Can you work these out from the model? Positions are in its coordinate system, mm. A direction names the side the tool comes from. Give positions to 0.01 mm unless a question says otherwise; leave off trailing zeros. Loops run counter-clockwise (first coordinate to the right, second up) from the corner with the lowest first, then second, coordinate; pieces in that order, holes last. Notation, with made-up numbers: (-36, 54) - (14, 54) arc R13 ccw to (14, 72) - close; hole circle Ø8 at (17.25, 53.5). An arc over 180 degrees is marked (long way). Write item = value, one per line.
from build123d import *

# Parameters (mm, degrees)
EXTRUDE_1_DEPTH        = 16
EXTRUDE_2_DEPTH        = 12
EXTRUDE_3_DEPTH        = 20
CUT_EXTRUDE_START      = -7
CUT_EXTRUDE_1_DEPTH    = 7
SKETCH_6_R             = 10
CUT_EXTRUDE_2_DEPTH    = 71.149839629
SKETCH_7_R             = 14
CUT_EXTRUDE_3_DEPTH    = 8
HOLE_WIZARD_M8_1_D     = 6.8
HOLE_WIZARD_M8_1_DEPTH = 16.25
HOLE_WIZARD_M8_1_TIP   = 2.042926105
CUT_EXTRUDE_4_DEPTH    = 84.868945385
FILLET_3_R             = 2
FILLET_6_R             = 5


with BuildPart() as part:
    # 草图1 → 凸台-拉伸1 (new body)
    with BuildSketch(Plane(origin=(0, 0, 0), x_dir=(1, 0, 0), z_dir=(0, 1, 0))):
        with BuildLine():
            Line((40, 5), (-40, 5))
            Line((-40, 5), (-40, 0))
            ThreePointArc((-40, 0), (0, -40), (40, 0))
            Line((40, 0), (40, 5))
        make_face()
    extrude(amount=EXTRUDE_1_DEPTH)

    # 草图3 → 凸台-拉伸2 (add)
    with BuildSketch(Plane(origin=(0, 16, 0), x_dir=(1, 0, 0), z_dir=(0, 1, 0))):
        with BuildLine():
            Line((-24, 5), (-24, 0))
            ThreePointArc((-24, 0), (0, -24), (24, 0))
            Line((24, 0), (24, 5))
            Line((24, 5), (-24, 5))
        make_face()
    extrude(amount=EXTRUDE_2_DEPTH)

    # 草图4 → 凸台-拉伸3 (add)
    with BuildSketch(Plane(origin=(0, 0, -5), x_dir=(-1, 0, 0), z_dir=(0, 0, -1))):
        with BuildLine():
            Line((-45, 23), (-45, -8))
            Line((-45, -8), (-40, -8))
            Line((-40, -8), (-40, 0))
            Line((-40, 0), (40, 0))
            Line((40, 0), (40, -8))
            Line((40, -8), (45, -8))
            Line((45, -8), (45, 23))
            ThreePointArc((45, 23), (43.535533906, 26.535533906), (40, 28))
            Line((40, 28), (-40, 28))
            ThreePointArc((-40, 28), (-43.535533906, 26.535533906), (-45, 23))
        make_face()
    extrude(amount=EXTRUDE_3_DEPTH)

    # 草图5 → 切除-拉伸1 (cut)
    with BuildSketch(Plane(origin=(0, 0, -25), x_dir=(-1, 0, 0), z_dir=(0, 0, -1)).offset(CUT_EXTRUDE_START)):
        with BuildLine():
            Line((-45, 8), (45, 8))
            Line((45, 8), (45, 23))
            ThreePointArc((45, 23), (43.535533906, 26.535533906), (40, 28))
            Line((40, 28), (-40, 28))
            ThreePointArc((-40, 28), (-43.535533906, 26.535533906), (-45, 23))
            Line((-45, 23), (-45, 8))
        make_face()
    extrude(amount=CUT_EXTRUDE_1_DEPTH, mode=Mode.SUBTRACT)

    # 草图6 → 切除-拉伸2 (cut, through all)
    with BuildSketch(Plane(origin=(0, 28, 0), x_dir=(1, 0, 0), z_dir=(0, 1, 0))):
        with Locations(Location((0, 0, 0), (0, 0, 270))):
            Circle(SKETCH_6_R)
    extrude(amount=-CUT_EXTRUDE_2_DEPTH, mode=Mode.SUBTRACT)

    # 草图7 → 切除-拉伸3 (cut)
    with BuildSketch(Plane(origin=(0, 28, 0), x_dir=(1, 0, 0), z_dir=(0, 1, 0))):
        with Locations(Location((0, 0, 0), (0, 0, 270))):
            Circle(SKETCH_7_R)
    extrude(amount=-CUT_EXTRUDE_3_DEPTH, mode=Mode.SUBTRACT)

    # M8 螺纹孔1
    with Locations(Plane(origin=(0, 0, -18), x_dir=(-1, 0, 0), z_dir=(0, 0, -1))):
        with Locations((-20, 19), (20, 19)):
            Hole(HOLE_WIZARD_M8_1_D / 2, depth=HOLE_WIZARD_M8_1_DEPTH)
            with Locations((0, 0, -(HOLE_WIZARD_M8_1_DEPTH + HOLE_WIZARD_M8_1_TIP / 2))):  # 118° drill point
                Cone(0, HOLE_WIZARD_M8_1_D / 2, HOLE_WIZARD_M8_1_TIP, mode=Mode.SUBTRACT)

    # 草图12 → 切除-拉伸4 (cut, through all)
    with BuildSketch(Plane(origin=(0, 0, -25), x_dir=(-1, 0, 0), z_dir=(0, 0, -1))):
        Polygon((-38.585786438, 0), (-40, 1.414213562), (-41.414213562, 0), (-40, -1.414213562), (-40, 0), align=None)
    cut_extrude_4 = extrude(amount=-CUT_EXTRUDE_4_DEPTH, mode=Mode.SUBTRACT)

    # 镜向1: 切除-拉伸4 across plane
    add(cut_extrude_4.mirror(Plane(origin=(0, 0, 0), x_dir=(0, 0, 1), z_dir=(1, 0, 0))), mode=Mode.SUBTRACT)

    # 圆角3
    fillet_3_edges = [part.edges().sort_by_distance(p)[0] for p in [
        (40, 16, -2.5),
        (0, 16, 40),
        (-40, 16, -2.5),
    ]]
    fillet(fillet_3_edges, radius=FILLET_3_R)

    # 圆角6
    fillet_6_edges = [part.edges().sort_by_distance(p)[0] for p in [
        (-24, 16, -2.5),
        (24, 16, -2.5),
        (-24, 22, -5),
        (24, 22, -5),
        (0, 16, 24),
    ]]
    fillet(fillet_6_edges, radius=FILLET_6_R - 0.0001)  # a hair under: the kernel refuses the full size


solid = part.part
Q1. Imagine slicing it at C-C, the plane x = 0. Write out the boundary of the cut face in (y, z).
Output:
outline = (0, -25) - (8, -25) - (8, -18) - (28, -18) - (28, -14) - (20, -14) - (20, -10) - (0, -10) - close; (0, 10) - (20, 10) - (20, 14) - (28, 14) - (28, 24) - (21, 24) arc R5 cw to (16, 29) - (16, 38) arc R2 ccw to (14, 40) - (0, 40) - close
Q2. Imagine slicing it at B-B, the plane y = 5.5. Write out the boundary of the cut face in (x, z).
Output:
outline = (-45, -25) - (45, -25) - (45, -5) - (40, -5) - (40, 0) arc R40 ccw to (-40, 0) - (-40, -5) - (-45, -5) - close; hole circle Ø20 at (0, 0)
Q3. For pin 1 (3.5 mm diameter, centred on x = 5.5, z = -22, fed in from +Y); pin 2 (5.5 mm diameter, centred on x = -20, y = 19, fed in from -Z); pin 3 (4 mm diameter, centred on x = 2, y = 7, fed in from +Z); pin 4 (16 mm diameter, centred on x = 0, z = 0, fed in from +Y), each with a flat end and sliding along its axis, tell me the tip position at first contact or that it passes through.
Output:
pin_1 = 8
pin_2 = -1.36
pin_3 = 40
pin_4 = through
Q4. I need wall thicknesses on L1, parallel to X at y = 23.5, z = 0; L2, parallel to X at y = -2, z = -11.5; L3, parallel to X at y = 0.5, z = -16.5. Which ranges of each line are inside material? Lowest first, please.
Output:
L1 = -24 to -14, 14 to 24
L2 = -45 to -40, 40 to 45
L3 = -45 to -40.91, -39.09 to 39.09, 40.91 to 45
Q5. Imagine slicing it at D-D, the plane y = -5. Write out the boundary of the cut face in (x, z).
Output:
outline = (-45, -25) - (-40, -25) - (-40, -5) - (-45, -5) - close; (40, -25) - (45, -25) - (45, -5) - (40, -5) - close
Q6. Which directions (+Z, -Z, +X, -X, +Y, -Y) give clear straight access to the entire face, cutting with the end or side of a thin tool? Please do faces 4 (the cylindrical face through (-0.528, 24.451, 23.994)), 5 (the flat face through (-40, 8, -3)), 6 (the flat face through (41, 14, -5)).
Output:
face_4 = +Z, +Y
face_5 = +Z, -X, +Y, -Y
face_6 = +Z, +X, +Y
Q7. We'd pull the mould along Z, two halves only. Please class faces 1 (the flat face through (9, 0, 8)), 2 (the cylindrical face through (-13.67, 24.06, -3.03)), 3 (the cylindrical face through (-26, 23, -4)): released by +Z, released by -Z, zero draft, split by the parting line, or undercut.
Output:
face_1 = zero draft
face_2 = undercut
face_3 = released by +Z
Q8. Imagine slicing it at A-A, the plane z = -7. Write out the boundary of the cut face in (x, y), then the cut area to 3 significant figures.
Output:
outline = (-45, -8) - (-40, -8) - (-40, -1.41) - (-41.41, 0) - (-40, 1.41) - (-38.59, 0) - (-7.14, 0) - (-7.14, 20) - (-12.12, 20) - (-12.12, 28) - (-40, 28) arc R5 ccw to (-45, 23) - close; (7.14, 0) - (38.59, 0) - (40, 1.41) - (41.41, 0) - (40, -1.41) - (40, -8) - (45, -8) - (45, 23) arc R5 ccw to (40, 28) - (12.12, 28) - (12.12, 20) - (7.14, 20) - close; hole circle Ø6.8 at (-20, 19); hole circle Ø6.8 at (20, 19)
area = 2,030 mm2
